Autodesk Inventor part; units mm, degrees
ref_plane "YZ Plane" through (0, 0, 0) normal (1, 0, 0) x (0, 1, 0)
ref_plane "XZ Plane" through (0, 0, 0) normal (0, 1, 0) x (-1, 0, 0)
ref_plane "XY Plane" through (0, 0, 0) normal (0, 0, 1) x (1, 0, 0)
sketch "草图1" plane through (0, 0, 0) normal (0, 0, 1) x (1, 0, 0)
  circle A0 centre (0, 0) radius 10
  dimension "d0" = 20
extrude "拉伸1" add sketch "草图1" along normal blind 5
sketch "草图2" plane through (0, 0, 5) normal (0, 0, 1) x (1, 0, 0)
  circle A0 centre (0, 0) radius 2.5
  dimension "d3" = 5
extrude "拉伸2" add sketch "草图2" along normal blind 27
thread "螺纹1"
chamfer "倒角1" distance 0.25 angle 45 1 edges at (-2.5, 0, 32)
properties part number "刀轴带动盘连杆固定螺丝"
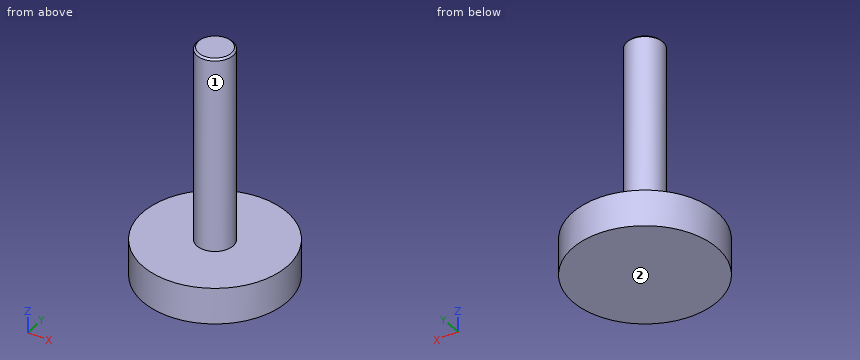
Read the model definition and answer for the solid it produces. Units are mm, in the model's axes. Face numbers are marked on the shaded views. A direction names the side the tool comes from. Give positions to 0.01 mm unless a question says otherwise; leave off trailing zeros. Write each loop counter-clockwise with the first axis right and the second up, starting at its lowest first coordinate (ties: lowest second). Pieces come first, ordered by that corner, then holes. Notation, with made-up numbers: M 7,82.5 L 44,82.5 A33 ccw 44,112.5 Z; hole C 31.25,-24.75 d2. An arc over 180 degrees is marked long. One line per item, written item: value. Start each with the question number.
(1) Find section D-D (x = 6.75). Determine the outline of the cut face in (y, z).
(2) Find section A-A (y = 0). Determine the outline of the cut face in (x, z).
(3) Find section C-C (z = 4). Determine the outline of the cut face in (x, y), plus the area to 3 significant figures.
(4) Find the intervals of material crossed by line 1 (Z direction, x = 7.5, y = -5.25); line 2 (Y direction, x = -1.5, z = 26), in increasing order.
(5) Flat-ended cylindrical pins translate along their axes: pin 1 Ø8 at (y, z) = (7, 5.5) entering from +X; pin 2 Ø1 at (x, y) = (1.5, 4) entering from +Z; pin 3 Ø5 at (x, z) = (-2.5, 20) entering from +Y; pin 4 Ø5 at (y, z) = (5.5, 22) entering from +X. Find the tip coordinate at first contact, or state that the pin passes through.
(6) A tool of negligible diameter and unlimited length cuts with its end or side. For the marked faces 1 and 2, from which of +Z, -Z, +X, -X, +Y, -Y can it reach the whole face along a straight path? Write none if from no direction.
Results below:
1. outline: M -7.38,0 L 7.38,0 L 7.38,5 L -7.38,5 Z
2. outline: M -10,0 L 10,0 L 10,5 L 2.5,5 L 2.5,31.75 L 2.25,32 L -2.25,32 L -2.5,31.75 L -2.5,5 L -10,5 Z
3. outline: C 0,0 d20
3. area: 314 mm^2
4. line 1: z = 0 to 5
4. line 2: y = -2 to 2
5. pin 1: stops at x = 9.53
5. pin 2: stops at z = 5
5. pin 3: stops at y = 2.5
5. pin 4: passes through
6. face 1: +Z
6. face 2: -Z, +X, -X, +Y, -Y
